Verification items for the finished model (mm, model axes). Coordinates: 2 decimals unless noted, no trailing zeros. Loops run counter-clockwise (first coordinate to the right, second up) from the corner with the lowest first, then second, coordinate; pieces in that order, holes last. Notation, with made-up numbers: (83, 87.5) -> (129, 87.5) arc R27 ccw to (129, 121.5) -> close; hole circle Ø5 at (-22, -7.75). An arc over 180 degrees is marked (long way). Answer as a JSON object with one key per item and string values. Group by question number.
Q1. Cross-section at C-C on y = -4.75. Record the boundary of the cut face in (x, z), and give its area (3 significant figures).
Q2. Cross-section at B-B on x = -2.5. Record the boundary of the cut face in (y, z).
Q3. Cross-section at A-A on x = 6. Record the boundary of the cut face in (y, z).
Q4. Scan lines: L1, parallel to Y at x = -6, z = 1.55; L2, parallel to Z at x = 10.5, y = -4.5; L3, parallel to X at y = 2.25, z = -1.5. Record each from-to range of solid material in increasing order.
Q5. Gauge pin test, flat ends, axial feed: pin 1 Ø1.5 at (x, y) = (6, 0) entering from +Z; pin 2 Ø8 at (x, y) = (1.5, 2) entering from -Z. Record the tip position at first contact, or that the pin passes through.
```python
from build123d import *

# Parameters (mm, degrees)
SKETCH1_W           = 32
SKETCH1_H           = 16
SKETCH1_R           = 1.25
BOSS_EXTRUDE1_DEPTH = 2
SKETCH2_W           = 2
SKETCH2_H           = 6
BOSS_EXTRUDE2_DEPTH = 5
BOSS_EXTRUDE2_TAPER = 5
FILLET1_R           = 1.5


with BuildPart() as part:
    # Sketch1 → Boss-Extrude1 (new body)
    with BuildSketch(Plane.XY):
        Rectangle(SKETCH1_W, SKETCH1_H)
        with Locations((6, 0)):
            Circle(SKETCH1_R, mode=Mode.SUBTRACT)
        with Locations((-6, 0)):
            Circle(SKETCH1_R, mode=Mode.SUBTRACT)
    extrude(amount=BOSS_EXTRUDE1_DEPTH)

    # Sketch2 → Boss-Extrude2 (add)
    with BuildSketch(Plane(origin=(0, 0, 0), x_dir=(-1, 0, 0), z_dir=(0, 0, -1))):
        with Locations((-13.5, 0)):
            Rectangle(SKETCH2_W, SKETCH2_H)
        with Locations((13.5, 0)):
            Rectangle(SKETCH2_W, SKETCH2_H)
    extrude(amount=BOSS_EXTRUDE2_DEPTH, taper=BOSS_EXTRUDE2_TAPER)

    # Fillet1
    fillet1_edges = [part.edges().sort_by_distance(p)[0] for p in [
        (-16, 8, 1),
        (16, 8, 1),
        (16, -8, 1),
        (-16, -8, 1),
    ]]
    fillet(fillet1_edges, radius=FILLET1_R)


solid = part.part
```
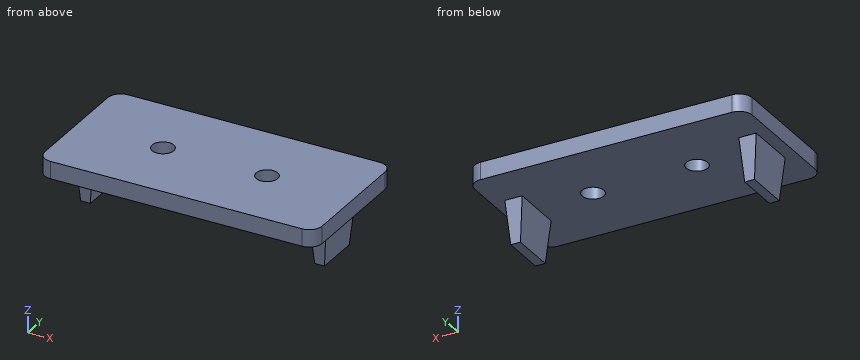
Computed values:
{
 "1": {"outline": "(-16, 0) -> (16, 0) -> (16, 2) -> (-16, 2) -> close", "area": "64.0 mm²"},
 "2": {"outline": "(-8, 0) -> (8, 0) -> (8, 2) -> (-8, 2) -> close"},
 "3": {"outline": "(-8, 0) -> (-1.25, 0) -> (-1.25, 2) -> (-8, 2) -> close; (1.25, 0) -> (8, 0) -> (8, 2) -> (1.25, 2) -> close"},
 "4": {"L1": "y = -8 to -1.25, 1.25 to 8", "L2": "z = 0 to 2", "L3": "x = -14.37 to -12.63, 12.63 to 14.37"},
 "5": {"pin 1": "passes through", "pin 2": "stops at z = 0"}
}
